The model under review builds one solid part; all positions refer to its coordinate system, in mm. Coordinates: 2 decimals unless noted, no trailing zeros. Loops run counter-clockwise (first coordinate to the right, second up) from the corner with the lowest first, then second, coordinate; pieces in that order, holes last. Notation, with made-up numbers: M -30,51 L 28,51 A13 cw 28,75 Z; hole C 35.25,47 d5. An arc over 180 degrees is marked long. Return JSON: item names as keys, results as strings.
```python
from build123d import *

# Parameters (mm, degrees)
SKETCH_1_W      = 120
SKETCH_1_H      = 20
SKETCH_1_R      = 1.6
EXTRUDE_1_DEPTH = 2
FILLET_1_R      = 4


with BuildPart() as part:
    # 草图1 → 凸台-拉伸1 (new body)
    with BuildSketch(Plane(origin=(0, 0, 0), x_dir=(1, 0, 0), z_dir=(0, 1, 0))):
        Rectangle(SKETCH_1_W, SKETCH_1_H)
        with Locations(Location((16, 0, 0), (0, 0, 270))):
            Circle(SKETCH_1_R, mode=Mode.SUBTRACT)
        with Locations(Location((-16, 0, 0), (0, 0, 270))):
            Circle(SKETCH_1_R, mode=Mode.SUBTRACT)
        with Locations(Location((36, 0, 0), (0, 0, 270))):
            Circle(SKETCH_1_R, mode=Mode.SUBTRACT)
        with Locations(Location((56, 0, 0), (0, 0, 270))):
            Circle(SKETCH_1_R, mode=Mode.SUBTRACT)
        with Locations(Location((-36, 0, 0), (0, 0, 270))):
            Circle(SKETCH_1_R, mode=Mode.SUBTRACT)
        with Locations(Location((-56, 0, 0), (0, 0, 270))):
            Circle(SKETCH_1_R, mode=Mode.SUBTRACT)
    extrude(amount=EXTRUDE_1_DEPTH)

    # 圆角1
    fillet_1_edges = [part.edges().sort_by_distance(p)[0] for p in [
        (60, 1, 10),
        (-60, 1, 10),
        (-60, 1, -10),
        (60, 1, -10),
    ]]
    fillet(fillet_1_edges, radius=FILLET_1_R)


solid = part.part
```
1. The part is to be moulded in two halves that separate along X. For faces 1 (the face through (-58.859, 1.014, 8.797)), 2 (the face through (-14.414, 0.986, -0.208)), 3 (the face through (-1, 1, -10)), 4 (the face through (34.58, 0.99, 0.74)), say which applies: released by +X, released by -X, zero draft, split by the parting line, or undercut.
Check values:
{"face 1": "released by -X", "face 2": "undercut", "face 3": "zero draft", "face 4": "undercut"}
2. Add section C-C on z = 0.5. Give the boundary of the cut face in (x, y), plus the area to 3 significant figures.
Check values:
{"outline": "M -60,0 L -57.52,0 L -57.52,2 L -60,2 Z; M -54.48,0 L -37.52,0 L -37.52,2 L -54.48,2 Z; M -34.48,0 L -17.52,0 L -17.52,2 L -34.48,2 Z; M -14.48,0 L 14.48,0 L 14.48,2 L -14.48,2 Z; M 17.52,0 L 34.48,0 L 34.48,2 L 17.52,2 Z; M 37.52,0 L 54.48,0 L 54.48,2 L 37.52,2 Z; M 57.52,0 L 60,0 L 60,2 L 57.52,2 Z", "area": "204 mm²"}
3. To check wall thickness, follow line 1 (X direction, y = 1.75, z = 8.75); line 2 (X direction, y = 0.45, z = 7). State the ranges of each line that lie inside material, in increasing order.
Check values:
{"line 1": "-58.9 to 58.9", "line 2": "-59.87 to 59.87"}
4. Add section B-B on x = -16. Give the boundary of the cut face in (y, z).
Check values:
{"outline": "M 0,-10 L 2,-10 L 2,-1.6 L 0,-1.6 Z; M 0,1.6 L 2,1.6 L 2,10 L 0,10 Z"}
5. Insertion check: pin 1 Ø10 at (x, z) = (34, -2) entering from -Y. The pin has a flat end and moves straight along its axis. Give the tip position at first contact, or say it passes through.
Check values:
{"pin 1": "y = 0"}
6. Add section A-A on y = 1.4. Give the boundary of the cut face in (x, z), plus the area to 3 significant figures.
Check values:
{"outline": "M -60,-6 A4 ccw -56,-10 L 56,-10 A4 ccw 60,-6 L 60,6 A4 ccw 56,10 L -56,10 A4 ccw -60,6 Z; hole C -56,0 d3.2; hole C -36,0 d3.2; hole C -16,0 d3.2; hole C 16,0 d3.2; hole C 36,0 d3.2; hole C 56,0 d3.2", "area": "2,340 mm²"}
